```python
from build123d import *

# Parameters (mm, degrees)
SKETCH_1_W          = 15
SKETCH_1_H          = 10
SKETCH_1_W_2        = 12.6
SKETCH_1_H_2        = 7.6
EXTRUDE_1_DEPTH     = 110
SKETCH_2_R          = 1.6
CUT_EXTRUDE_1_DEPTH = 100
SKETCH_3_R          = 1.6
CUT_EXTRUDE_2_DEPTH = 15
SKETCH_5_W          = 15
SKETCH_5_H          = 10
CUT_EXTRUDE_4_DEPTH = 14.5
SKETCH_6_R          = 1.6
CUT_EXTRUDE_5_DEPTH = 15
SKETCH_7_R          = 1.6
CUT_EXTRUDE_6_DEPTH = 10


with BuildPart() as part:
    # ｽｹｯﾁ1 → ﾎﾞｽ - 押し出し1 (new, symmetric)
    with BuildSketch(Plane(origin=(0, 0, 0), x_dir=(1, 0, 0), z_dir=(0, 1, 0))):
        Rectangle(SKETCH_1_W, SKETCH_1_H)
        Rectangle(SKETCH_1_W_2, SKETCH_1_H_2, mode=Mode.SUBTRACT)
    extrude(amount=EXTRUDE_1_DEPTH, both=True)

    # ｽｹｯﾁ2 → ｶｯﾄ - 押し出し1 (cut)
    with BuildSketch(Plane(origin=(0, 0, -5), x_dir=(-1, 0, 0), z_dir=(0, 0, -1))):
        with Locations((0, -85)):
            Circle(SKETCH_2_R)
        with Locations((0, -105)):
            Circle(SKETCH_2_R)
    extrude(amount=-CUT_EXTRUDE_1_DEPTH, mode=Mode.SUBTRACT)

    # ｽｹｯﾁ3 → ｶｯﾄ - 押し出し2 (cut)
    with BuildSketch(Plane(origin=(7.5, 0, 0), x_dir=(0, 0, -1), z_dir=(1, 0, 0))):
        with Locations((0, -34)):
            Circle(SKETCH_3_R)
        with Locations((0, -74)):
            Circle(SKETCH_3_R)
    extrude(amount=-CUT_EXTRUDE_2_DEPTH, mode=Mode.SUBTRACT)

    # ｽｹｯﾁ5 → ｶｯﾄ - 押し出し4 (cut)
    with BuildSketch(Plane(origin=(0, 110, 0), x_dir=(1, 0, 0), z_dir=(0, 1, 0))):
        Rectangle(SKETCH_5_W, SKETCH_5_H)
    extrude(amount=-CUT_EXTRUDE_4_DEPTH, mode=Mode.SUBTRACT)

    # ｽｹｯﾁ6 → ｶｯﾄ - 押し出し5 (cut)
    with BuildSketch(Plane(origin=(0, 0, -5), x_dir=(-1, 0, 0), z_dir=(0, 0, -1))):
        with Locations((0, 90.5)):
            Circle(SKETCH_6_R)
        with Locations((0, 76.66)):
            Circle(SKETCH_6_R)
        with Locations((0, 56.66)):
            Circle(SKETCH_6_R)
    extrude(amount=-CUT_EXTRUDE_5_DEPTH, mode=Mode.SUBTRACT)

    # ｽｹｯﾁ7 → ｶｯﾄ - 押し出し6 (cut)
    with BuildSketch(Plane(origin=(0, 0, -5), x_dir=(-1, 0, 0), z_dir=(0, 0, -1))):
        with Locations((0, 9.6)):
            Circle(SKETCH_7_R)
        with Locations((0, 29.6)):
            Circle(SKETCH_7_R)
    extrude(amount=-CUT_EXTRUDE_6_DEPTH, mode=Mode.SUBTRACT)


solid = part.part
```
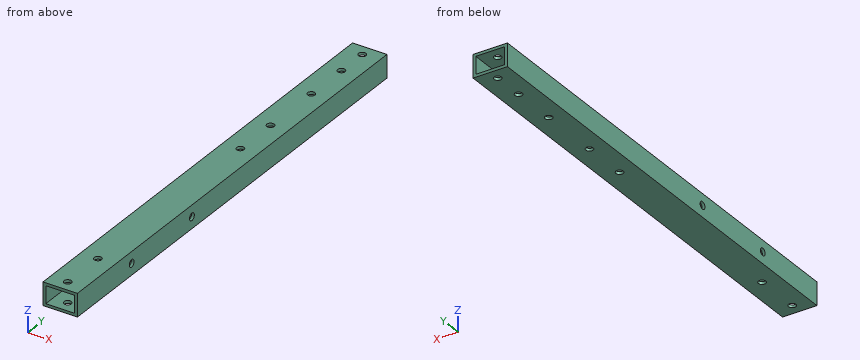
Geometry check sheet. Reference: the model listing, model coordinates, mm. Give positions to 0.01 mm unless a question says otherwise; leave off trailing zeros. Order: outer loops, then holes, each group sorted by start corner. A loop starts at its lowest first (then second) coordinate and runs counter-clockwise, first axis right, second up.
1. Section check C-C, the plane z = 0. Enter the section's corners in (x, y), and give its area (3 significant figures).
2. Section check B-B, the plane y = -40.5. Enter the section's corners in (x, z).
3. Thickness scan on L1, parallel to Z at x = -4, y = -53; L2, parallel to X at y = -44.5, z = 1.75; L3, parallel to X at y = -105, z = -4.3. Record the ranges inside material, lowest first.
4. Section check A-A, the plane x = 4. Enter the section's corners in (y, z).
Values follow:
1. outline: (-7.5, -110) - (-6.3, -110) - (-6.3, -75.6) - (-7.5, -75.6) - close; (-7.5, -72.4) - (-6.3, -72.4) - (-6.3, -35.6) - (-7.5, -35.6) - close; (-7.5, -32.4) - (-6.3, -32.4) - (-6.3, 95.5) - (-7.5, 95.5) - close; (6.3, -110) - (7.5, -110) - (7.5, -75.6) - (6.3, -75.6) - close; (6.3, -72.4) - (7.5, -72.4) - (7.5, -35.6) - (6.3, -35.6) - close; (6.3, -32.4) - (7.5, -32.4) - (7.5, 95.5) - (6.3, 95.5) - close
1. area: 478 mm2
2. outline: (-7.5, -5) - (7.5, -5) - (7.5, 5) - (-7.5, 5) - close; hole (-6.3, -3.8) - (6.3, -3.8) - (6.3, 3.8) - (-6.3, 3.8) - close
3. L1: z = -5 to -3.8, 3.8 to 5
3. L2: x = -7.5 to -6.3, 6.3 to 7.5
3. L3: x = -7.5 to -1.6, 1.6 to 7.5
4. outline: (-110, -5) - (95.5, -5) - (95.5, -3.8) - (-110, -3.8) - close; (-110, 3.8) - (95.5, 3.8) - (95.5, 5) - (-110, 5) - close
